CAD build for the part. Positions are in the model's coordinates, mm. Face numbers are marked on the shaded views. A direction names the side the tool comes from. Round coordinates to 2 decimals unless told otherwise and drop trailing zeros. Order: outer loops, then holes, each group sorted by start corner. A loop starts at its lowest first (then second) coordinate and runs counter-clockwise, first axis right, second up. Notation, with made-up numbers: (-8, 16.5) -> (51, 16.5) arc R17 cw to (51, 31.5) -> close; hole circle Ø1 at (65.25, 22.25). An arc over 180 degrees is marked (long way). Return JSON: item names as keys, results as strings. Group by question number.
Q1. Mould opens along Y. For the marked faces 1, 2, 3 and 4 say: +Y half, -Y half, draft (parallel to the pull), parting line (faces both ways), or undercut.
Q2. Cut at A-A (x = 44.45). Write the cut outline in (y, z) (1 decimal), then the cut area to 3 significant figures.
Q3. Cut at D-D (x = -25). Write the cut outline in (y, z).
Q4. Cut at C-C (x = -6.35). Write the cut outline in (y, z).
Q5. Flat gauge pins, fed straight in: pin 1 (6 mm diameter, centred on y = 2.5, z = 9.5, fed in from +X); pin 2 (5.5 mm diameter, centred on x = 30.22, y = 15.488, fed in from +Z); pin 3 (5 mm diameter, centred on x = -19, y = 1.5, fed in from -Z); pin 4 (1.1 mm diameter, centred on x = -40, y = -14.5, fed in from +Z). Where does each tip first touch, or does it go through?
Q6. Probe line 1 along X through (y, z) = (27.5, 17.78); line 2 along Z through (x, y) = (44.45, 16); line 3 along Y through (x, z) = (49, 5.5). List the from-to ranges inside material, lowest first.
Q7. Cut at B-B (y = 33). Count the separate pieces of the cut face and the enclosed holes in it, then the cut area to 3 significant figures.
Q8. Which spindle directions (+Z, -Z, +X, -X, +Y, -Y) get a long thin tool onto all of the face, cutting with end or side? Do the marked faces 5, 6, 7 and 8. Say none if no direction does.
from build123d import *

# Parameters (mm, degrees)
SKETCH1_W           = 114.3
SKETCH1_H           = 76.2
BOSS_EXTRUDE1_DEPTH = 25.4
CUT_EXTRUDE1_DEPTH  = 6.477
CUT_EXTRUDE2_DEPTH  = 18.923
SKETCH4_W           = 20.574
SKETCH4_H           = 25.4
CUT_EXTRUDE3_DEPTH  = 6.35
CUT_EXTRUDE4_START  = -25.4
CUT_EXTRUDE4_DEPTH  = 25.4
CUT_EXTRUDE5_START  = -25.4
SKETCH6_R           = 1.75
SKETCH6_R_2         = 11.1125
CUT_EXTRUDE5_DEPTH  = 25.4
SKETCH8_R           = 3.175
CUT_EXTRUDE6_DEPTH  = 12.7
FILLET1_R           = 3.175
CUT_EXTRUDE7_START  = -76.2
SKETCH9_R           = 2.5796875
CUT_EXTRUDE7_DEPTH  = 76.2
SKETCH10_R          = 4.7625
CUT_EXTRUDE8_DEPTH  = 15.875
SKETCH11_R          = 4.7625
CUT_EXTRUDE9_DEPTH  = 15.875
FILLET2_R           = 3.175
SKETCH12_R          = 2.032
CUT_EXTRUDE10_DEPTH = 12.446
SKETCH13_R          = 1.35255
CUT_EXTRUDE11_DEPTH = 12.7
SKETCH14_R          = 1.143
CUT_EXTRUDE12_DEPTH = 12.7


with BuildPart() as part:
    # Sketch1 → Boss-Extrude1 (new body)
    with BuildSketch(Plane.XY):
        Rectangle(SKETCH1_W, SKETCH1_H)
    extrude(amount=BOSS_EXTRUDE1_DEPTH)

    # Sketch2 → Cut-Extrude1 (cut)
    with BuildSketch(Plane.XY.offset(25.4)):
        with BuildLine():
            Line((-52.959, 5.939202219), (-52.959, -5.939202219))
            ThreePointArc((-52.959, -5.939202219), (-22.098, 0), (-52.959, 5.939202219))
        make_face()
    extrude(amount=-CUT_EXTRUDE1_DEPTH, mode=Mode.SUBTRACT)

    # Sketch3 → Cut-Extrude2 (cut)
    with BuildSketch(Plane.XY.offset(18.923)):
        with BuildLine():
            Line((-17.276835078, 12.319), (-28.067, 12.319))
            ThreePointArc((-28.067, 12.319), (-38.1, 15.887694924), (-48.133, 12.319))
            Line((-48.133, 12.319), (-57.15, 12.319))
            Line((-57.15, 12.319), (-57.15, -12.319))
            Line((-57.15, -12.319), (-48.133, -12.319))
            ThreePointArc((-48.133, -12.319), (-38.1, -15.887694924), (-28.067, -12.319))
            Line((-28.067, -12.319), (-17.276835078, -12.319))
            ThreePointArc((-17.276835078, -12.319), (-12.782632352, -12.236367648), (-12.7, -7.742164922))
            Line((-12.7, -7.742164922), (-12.7, 7.742164922))
            ThreePointArc((-12.7, 7.742164922), (-12.782632352, 12.236367648), (-17.276835078, 12.319))
        make_face()
    extrude(amount=-CUT_EXTRUDE2_DEPTH, mode=Mode.SUBTRACT)

    # Sketch4 → Cut-Extrude3 (cut)
    with BuildSketch(Plane(origin=(0, 38.1, 0), x_dir=(1, 0, 0), z_dir=(0, 1, 0))):
        with Locations((2.413, -12.7)):
            Rectangle(SKETCH4_W, SKETCH4_H)
    extrude(amount=-CUT_EXTRUDE3_DEPTH, mode=Mode.SUBTRACT)

    # Sketch5 → Cut-Extrude4 (cut)
    with BuildSketch(Plane(origin=(0, 0, 0), x_dir=(-1, 0, 0), z_dir=(0, 0, -1)).offset(CUT_EXTRUDE4_START)):
        with BuildLine():
            Line((-36.075066976, -12.827), (-57.15, -12.827))
            Line((-57.15, -12.827), (-57.15, 12.827))
            Line((-57.15, 12.827), (-36.075066976, 12.827))
            ThreePointArc((-36.075066976, 12.827), (-31.451098719, 12.871901281), (-31.496, 8.247933024))
            Line((-31.496, 8.247933024), (-31.496, -8.247933024))
            ThreePointArc((-31.496, -8.247933024), (-31.451098719, -12.871901281), (-36.075066976, -12.827))
        make_face()
    extrude(amount=CUT_EXTRUDE4_DEPTH, mode=Mode.SUBTRACT)

    # Sketch6 → Cut-Extrude5 (cut)
    with BuildSketch(Plane(origin=(0, 0, 0), x_dir=(-1, 0, 0), z_dir=(0, 0, -1)).offset(CUT_EXTRUDE5_START)):
        with Locations((0.768, 15.5)):
            Circle(SKETCH6_R)
        with Locations((0.768, -15.5)):
            Circle(SKETCH6_R)
        with Locations((-14.732, 0)):
            Circle(SKETCH6_R_2)
        with Locations((-30.22, -15.5)):
            Circle(SKETCH6_R)
        with Locations((-30.22, 15.488)):
            Circle(SKETCH6_R)
    extrude(amount=CUT_EXTRUDE5_DEPTH, mode=Mode.SUBTRACT)

    # Sketch8 → Cut-Extrude6 (cut)
    with BuildSketch(Plane.XY.offset(25.4)):
        with Locations((-0.768, -15.5)):
            Circle(SKETCH8_R)
        with Locations((-0.768, 15.5)):
            Circle(SKETCH8_R)
        with Locations((30.22, -15.5)):
            Circle(SKETCH8_R)
        with Locations((30.22, 15.488)):
            Circle(SKETCH8_R)
    extrude(amount=-CUT_EXTRUDE6_DEPTH, mode=Mode.SUBTRACT)

    # Fillet1
    fillet1_edges = [part.edges().sort_by_distance(p)[0] for p in [
        (-57.15, 38.1, 12.7),
        (57.15, 38.1, 12.7),
        (57.15, -38.1, 12.7),
        (-57.15, -38.1, 12.7),
        (57.15, -12.827, 12.7),
        (57.15, 12.827, 12.7),
    ]]
    fillet(fillet1_edges, radius=FILLET1_R)

    # Sketch9 → Cut-Extrude7 (cut)
    with BuildSketch(Plane(origin=(0, 38.1, 0), x_dir=(1, 0, 0), z_dir=(0, 1, 0)).offset(CUT_EXTRUDE7_START)):
        with Locations((44.45, -12.7)):
            Circle(SKETCH9_R)
    extrude(amount=CUT_EXTRUDE7_DEPTH, mode=Mode.SUBTRACT)

    # Sketch10 → Cut-Extrude8 (cut)
    with BuildSketch(Plane(origin=(0, 38.1, 0), x_dir=(1, 0, 0), z_dir=(0, 1, 0))):
        with Locations((44.45, -12.7)):
            Circle(SKETCH10_R)
    extrude(amount=-CUT_EXTRUDE8_DEPTH, mode=Mode.SUBTRACT)

    # Sketch11 → Cut-Extrude9 (cut)
    with BuildSketch(Plane.XZ.offset(38.1)):
        with Locations((44.45, 12.7)):
            Circle(SKETCH11_R)
    extrude(amount=-CUT_EXTRUDE9_DEPTH, mode=Mode.SUBTRACT)

    # Fillet2
    fillet2_edges = [part.edges().sort_by_distance(p)[0] for p in [
        (-17.276835078, 12.319, 9.4615),
        (-12.7, 7.742164922, 9.4615),
        (-12.7, -7.742164922, 9.4615),
        (-17.276835078, -12.319, 9.4615),
        (36.075066976, 12.827, 12.7),
        (31.496, 8.247933024, 12.7),
        (31.496, -8.247933024, 12.7),
        (36.075066976, -12.827, 12.7),
    ]]
    fillet(fillet2_edges, radius=FILLET2_R)

    # Sketch12 → Cut-Extrude10 (cut)
    with BuildSketch(Plane.XZ.offset(38.1)):
        with Locations((-6.35, 12.682334878)):
            Circle(SKETCH12_R)
    extrude(amount=-CUT_EXTRUDE10_DEPTH, mode=Mode.SUBTRACT)

    # Sketch13 → Cut-Extrude11 (cut)
    with BuildSketch(Plane.ZY.offset(57.15)):
        with Locations((12.7, 28.575)):
            Circle(SKETCH13_R)
        with Locations((12.7, -28.575)):
            Circle(SKETCH13_R)
    extrude(amount=-CUT_EXTRUDE11_DEPTH, mode=Mode.SUBTRACT)

    # Sketch14 → Cut-Extrude12 (cut)
    with BuildSketch(Plane(origin=(0, 31.75, 0), x_dir=(1, 0, 0), z_dir=(0, 1, 0))):
        with Locations((-2.54, -17.78)):
            Circle(SKETCH14_R)
        with Locations((7.366, -17.78)):
            Circle(SKETCH14_R)
    extrude(amount=-CUT_EXTRUDE12_DEPTH, mode=Mode.SUBTRACT)


solid = part.part
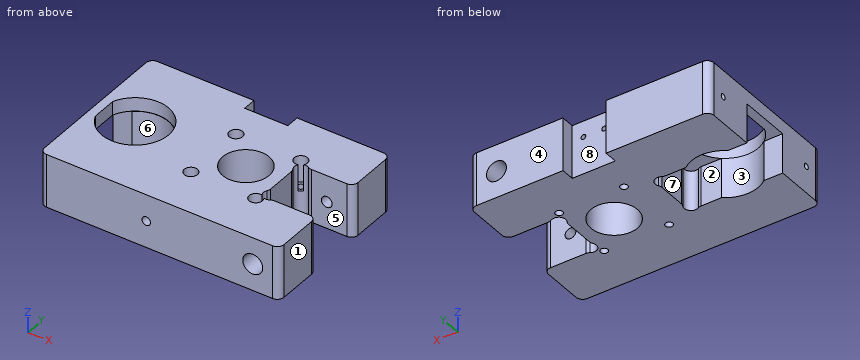
Solution:
{
 "1": {"face 1": "draft", "face 2": "undercut", "face 3": "undercut", "face 4": "+Y half"},
 "2": {"outline": "(-38.1, 0) -> (-12.8, 0) -> (-12.8, 10.1) -> (-22.2, 10.1) -> (-22.2, 7.9) -> (-38.1, 7.9) -> close; (-38.1, 17.5) -> (-22.2, 17.5) -> (-22.2, 15.3) -> (-12.8, 15.3) -> (-12.8, 25.4) -> (-38.1, 25.4) -> close; (12.8, 0) -> (38.1, 0) -> (38.1, 7.9) -> (22.2, 7.9) -> (22.2, 10.1) -> (12.8, 10.1) -> close; (12.8, 15.3) -> (22.2, 15.3) -> (22.2, 17.5) -> (38.1, 17.5) -> (38.1, 25.4) -> (12.8, 25.4) -> close", "area": "884 mm²"},
 "3": {"outline": "(-38.1, 0) -> (-12.32, 0) -> (-12.32, 18.92) -> (-9.19, 18.92) -> (-9.19, 25.4) -> (-38.1, 25.4) -> close; (9.19, 18.92) -> (12.32, 18.92) -> (12.32, 0) -> (38.1, 0) -> (38.1, 25.4) -> (9.19, 25.4) -> close"},
 "4": {"outline": "(-38.1, 0) -> (31.75, 0) -> (31.75, 25.4) -> (-38.1, 25.4) -> (-38.1, 14.71) -> (-25.65, 14.71) -> (-25.65, 10.65) -> (-38.1, 10.65) -> close"},
 "5": {"pin 1": "stops at x = 31.5", "pin 2": "stops at z = 12.7", "pin 3": "stops at z = 18.92", "pin 4": "passes through"},
 "6": {"line 1": "x = -57.15 to -3.68, -1.4 to 6.22, 8.51 to 57.15", "line 2": "z = 0 to 10.12, 15.28 to 25.4", "line 3": "y = -38.1 to -12.83, 12.83 to 38.1"},
 "7": {"separate pieces": "2", "enclosed holes": "1", "area": "2,310 mm²"},
 "8": {"face 5": "+Z, -Z, +X", "face 6": "+Z, -Z", "face 7": "-Z, -X", "face 8": "+Z, -Z, +Y"}
}
